Read the model definition and answer for the solid it produces. Units are mm, in the model's axes. A direction names the side the tool comes from. Coordinates: 2 decimals unless noted, no trailing zeros. Order: outer loops, then holes, each group sorted by start corner. A loop starts at its lowest first (then second) coordinate and runs counter-clockwise, first axis right, second up.
```python
from build123d import *

# Parameters (mm, degrees)
EXTRUDE_1_DEPTH     = 16.5
SKETCH_2_R          = 1.6
CUT_EXTRUDE_1_DEPTH = 6
SKETCH_3_R          = 1.6
CUT_EXTRUDE_2_DEPTH = 10
EXTRUDE_2_DEPTH     = 1
EXTRUDE_3_DEPTH     = 1


with BuildPart() as part:
    # 草图1 → 凸台-拉伸1 (new body)
    with BuildSketch(Plane(origin=(0, 0, 0), x_dir=(1, 0, 0), z_dir=(0, 1, 0))):
        Polygon((0, 0), (12, 0), (12, 16), (11, 16), (11, 1), (0, 1), align=None)
    extrude(amount=EXTRUDE_1_DEPTH)

    # 草图2 → 切除-拉伸1 (cut)
    with BuildSketch(Plane(origin=(12, 0, 0), x_dir=(0, 0, -1), z_dir=(1, 0, 0))):
        with Locations((12.5, 11.5)):
            Circle(SKETCH_2_R)
    extrude(amount=-CUT_EXTRUDE_1_DEPTH, mode=Mode.SUBTRACT)

    # 草图3 → 切除-拉伸2 (cut)
    with BuildSketch(Plane(origin=(0, 0, -1), x_dir=(-1, 0, 0), z_dir=(0, 0, -1))):
        with Locations((-3.5, 5)):
            Circle(SKETCH_3_R)
        with Locations((-3.5, 11.5)):
            Circle(SKETCH_3_R)
    extrude(amount=-CUT_EXTRUDE_2_DEPTH, mode=Mode.SUBTRACT)

    # 草图4 → 凸台-拉伸2 (add)
    with BuildSketch(Plane.XZ):
        Polygon((0, -1), (11, -1), (11, -16), align=None)
    extrude(amount=-EXTRUDE_2_DEPTH)

    # 草图5 → 凸台-拉伸3 (add)
    with BuildSketch(Plane(origin=(0, 16.5, 0), x_dir=(1, 0, 0), z_dir=(0, 1, 0))):
        Polygon((0, 1), (11, 1), (11, 16), align=None)
    extrude(amount=-EXTRUDE_3_DEPTH)


solid = part.part
```
1) A cutting plane is placed at B-B, the plane y = 11.5. Determine the outline of the cut face in (x, z).
A:
outline: (0, -1) - (1.9, -1) - (1.9, 0) - (0, 0) - close; (5.1, -1) - (11, -1) - (11, -10.9) - (12, -10.9) - (12, 0) - (5.1, 0) - close; (11, -16) - (12, -16) - (12, -14.1) - (11, -14.1) - close
2) A cutting plane is placed at A-A, the plane y = 5. Determine the outline of the cut face in (x, z).
A:
outline: (0, -1) - (1.9, -1) - (1.9, 0) - (0, 0) - close; (5.1, -1) - (11, -1) - (11, -16) - (12, -16) - (12, 0) - (5.1, 0) - close
3) Straight lines are drawn through the part: line 1 (Y direction, x = 3.5, z = -0.15); line 2 (Y direction, x = 7, z = -2.25); line 3 (X direction, y = 8.5, z = -2.25). For each, find the intervals that lie inside material, in ascending order.
A:
line 1: y = 0 to 3.4, 6.6 to 9.9, 13.1 to 16.5
line 2: y = 0 to 1, 15.5 to 16.5
line 3: x = 11 to 12
4) Flat-ended cylindrical pins translate along their axes: pin 1 Ø5.5 at (x, y) = (3.5, 6.5) entering from -Z; pin 2 Ø7 at (y, z) = (8.5, -11) entering from -X. Find the tip coordinate at first contact, or state that the pin passes through.
A:
pin 1: stops at z = -1
pin 2: stops at x = 11
5) A cutting plane is placed at D-D, the plane z = -11.75. Determine the outline of the cut face in (x, y), and give its area (3 significant figures).
A:
outline: (7.88, 0) - (12, 0) - (12, 10.09) - (11, 10.09) - (11, 1) - (7.88, 1) - close; (7.88, 15.5) - (11, 15.5) - (11, 12.91) - (12, 12.91) - (12, 16.5) - (7.88, 16.5) - close
area: 19.9 mm2
6) Determine the mould class of faces 1 (the flat face through (0, 8.1, -0.5)), 2 (the cylindrical face through (2.76, 3.58, -0.51)), 3 (the flat face through (6, 8, -1)) for opening direction X: pulls with the +X half, pulls with the -X half, needs draft (parallel to the pull), parting line crosses it, or undercut.
A:
face 1: pulls with the -X half
face 2: undercut
face 3: needs draft
7) Which of the six approach directions +Z, -Z, +X, -X, +Y, -Y give full straight-line access (tool end or side, diameter ignored) to faces 4 (the cylindrical face through (11.51, 11.57, -10.9)), 5 (the flat face through (11, 8, -9))?
A:
face 4: +X, -X
face 5: -Z, -X
8) A cutting plane is placed at C-C, the plane x = 2.25. Determine the outline of the cut face in (y, z), and give its area (3 significant figures).
A:
outline: (0, -4.07) - (1, -4.07) - (1, -1) - (4, -1) - (4, 0) - (0, 0) - close; (6, -1) - (10.5, -1) - (10.5, 0) - (6, 0) - close; (12.5, -1) - (15.5, -1) - (15.5, -4.07) - (16.5, -4.07) - (16.5, 0) - (12.5, 0) - close
area: 18.6 mm2
